Input: part model. Units: mm. Frame: model coordinates. A direction names the side the tool comes from. Round coordinates to 2 decimals unless told otherwise and drop trailing zeros. Loops run counter-clockwise (first coordinate to the right, second up) from the corner with the lowest first, then second, coordinate; pieces in that order, holes last. Notation, with made-up numbers: (32.25, 14) -> (89.25, 14) arc R14 cw to (89.25, 37) -> close; hole circle Ø7 at (29, 65). An arc over 180 degrees is marked (long way). Answer as a JSON object with one key per item and string values.
Autodesk Inventor part; units mm, degrees
ref_plane "YZ Plane" through (0, 0, 0) normal (1, 0, 0) x (0, 1, 0)
ref_plane "XY Plane" through (0, 0, 0) normal (0, 0, 1) x (1, 0, 0)
sketch "Sketch1" plane through (0, 0, 0) normal (0, 1, 0) x (-1, 0, 0)
  arc A0 (24.5855, 23.6396) -> (8.8578, 61.8356) centre (-39.8212, 19.4554) ccw
  arc A1 (8.8578, 61.8356) -> (-24.5592, 49.0787) centre (-2.8694, 42.4084) ccw
  arc A2 (-27.4284, -51.6159) -> (7.5457, -75.9974) centre (10.0017, -35.1993) ccw
  arc A3 (7.5457, -75.9974) -> (24.5855, 23.6396) centre (-254.8198, 20.1477) ccw
  arc A4 (21.8724, 23.5336) -> (7.0955, 59.7239) centre (-39.8212, 19.4554) ccw
  arc A5 (7.0955, 59.7239) -> (-21.8846, 48.5356) centre (-2.8694, 42.4084) ccw
  arc A6 (-21.8846, -56.1581) -> (5.7032, -73.1142) centre (10.0017, -35.1993) ccw
  arc A7 (5.7032, -73.1142) -> (21.8724, 23.5336) centre (-254.8198, 20.1477) ccw
  line L0 (-21.8846, 48.5356) -> (-21.8846, -56.1581)
  line L1 (-24.5592, 49.0787) -> (-27.4313, -51.6092)
  arc A8 (24.5855, 23.6396) -> (8.8578, 61.8356) centre (-39.8212, 19.4554) ccw
  arc A9 (8.8578, 61.8356) -> (-24.5592, 49.0787) centre (-2.8694, 42.4084) ccw
  arc A10 (-27.4313, -51.6092) -> (7.5457, -75.9974) centre (10.0017, -35.1993) ccw
  arc A11 (7.5457, -75.9974) -> (24.5855, 23.6396) centre (-254.8198, 20.1477) ccw
  line L2 (-24.5592, 49.0787) -> (-27.4313, -51.6092)
  point P0 (0, 0)
extrude "Extrusion1" add sketch "Sketch1" along normal blind 15.24
sketch "Sketch2" plane through (0, 0, 0) normal (0, 1, 0) x (-1, 0, 0)
  arc A0 (21.8724, 23.5336) -> (7.0955, 59.7239) centre (-39.8212, 19.4554) ccw
  arc A1 (5.7032, -73.1142) -> (21.8724, 23.5336) centre (-254.8198, 20.1477) ccw
  arc A2 (-21.8846, -56.1581) -> (5.7032, -73.1142) centre (10.0017, -35.1993) ccw
  line L0 (-21.8846, -56.1581) -> (-21.8846, 48.5356)
  arc A3 (7.0955, 59.7239) -> (-21.8846, 48.5356) centre (-2.8694, 42.4084) ccw
  arc A4 (20.2233, 23.4688) -> (6.03, 58.4313) centre (-39.8212, 19.4554) ccw
  arc A5 (6.03, 58.4313) -> (-20.235, 48.2707) centre (-2.8694, 42.4084) ccw
  line L1 (-20.235, 48.2707) -> (-20.235, -55.6586)
  arc A6 (-20.235, -55.6586) -> (4.5953, -71.3048) centre (10.0017, -35.1993) ccw
  arc A7 (4.5953, -71.3048) -> (20.2233, 23.4688) centre (-254.8198, 20.1477) ccw
  arc A8 (21.96, 23.537) -> (7.1522, 59.7924) centre (-39.8212, 19.4554) ccw
  arc A9 (7.1522, 59.7924) -> (-21.9723, 48.5494) centre (-2.8694, 42.4084) ccw
  line L2 (-21.9723, 48.5494) -> (-21.9723, -56.1844)
  arc A10 (-21.9723, -56.1844) -> (5.7624, -73.209) centre (10.0017, -35.1993) ccw
  arc A11 (5.7624, -73.209) -> (21.96, 23.537) centre (-254.8198, 20.1477) ccw
  point P0 (0, 0)
ref_plane "Work Plane2" through (0, 7.62, 0) normal (0, 1, 0) x (-1, 0, 0)
sketch "Sketch3" plane through (0, 7.62, 0) normal (0, 1, 0) x (-1, 0, 0)
  arc A0 (21.8724, 23.5336) -> (7.0955, 59.7239) centre (-39.8212, 19.4554) ccw
  arc A1 (5.7032, -73.1142) -> (21.8724, 23.5336) centre (-254.8198, 20.1477) ccw
  arc A2 (-21.8846, -56.1581) -> (5.7032, -73.1142) centre (10.0017, -35.1993) ccw
  arc A3 (5.7032, -73.1142) -> (21.8724, 23.5336) centre (-254.8198, 20.1477) ccw
  arc A4 (-21.8846, -56.1581) -> (5.7032, -73.1142) centre (10.0017, -35.1993) ccw
  line L0 (-21.8846, -56.1581) -> (-21.8846, 48.5356)
  arc A5 (7.0955, 59.7239) -> (-21.8846, 48.5356) centre (-2.8694, 42.4084) ccw
  arc A6 (21.8724, 23.5336) -> (7.0955, 59.7239) centre (-39.8212, 19.4554) ccw
  arc A7 (8.8578, 61.8356) -> (-24.5592, 49.0787) centre (-2.8694, 42.4084) ccw
  line L1 (-24.5592, 49.0787) -> (-27.4313, -51.6092)
  arc A8 (-27.4313, -51.6092) -> (7.5457, -75.9974) centre (10.0017, -35.1993) ccw
  arc A9 (7.5457, -75.9974) -> (24.5855, 23.6396) centre (-254.8198, 20.1477) ccw
  arc A10 (24.5855, 23.6396) -> (8.8578, 61.8356) centre (-39.8212, 19.4554) ccw
  arc A11 (20.0927, 23.4636) -> (5.7444, 58.5644) centre (-39.8212, 19.4554) ccw
  arc A12 (4.508, -71.1594) -> (20.0927, 23.4636) centre (-254.8198, 20.1477) ccw
  arc A13 (-20.3969, -55.1802) -> (4.508, -71.1594) centre (10.0017, -35.1993) ccw
  line L2 (-20.0973, 48.248) -> (-20.0973, -55.6163)
  arc A14 (-20.0973, -55.6163) -> (4.5033, -71.1517) centre (10.0017, -35.1993) ccw
  arc A15 (4.5033, -71.1517) -> (20.0858, 23.4633) centre (-254.8198, 20.1477) ccw
  arc A16 (20.0858, 23.4633) -> (5.9414, 58.323) centre (-39.8212, 19.4554) ccw
  arc A17 (5.9414, 58.323) -> (-20.0973, 48.248) centre (-2.8694, 42.4084) ccw
  arc A18 (21.9213, 23.5355) -> (7.1272, 59.7622) centre (-39.8212, 19.4554) ccw
  arc A19 (5.7363, -73.1672) -> (21.9213, 23.5355) centre (-254.8198, 20.1477) ccw
  arc A20 (-21.9336, -56.1728) -> (5.7363, -73.1672) centre (10.0017, -35.1993) ccw
  line L3 (-21.9336, -56.1728) -> (-21.9336, 48.5433)
  arc A21 (7.1272, 59.7622) -> (-21.9336, 48.5433) centre (-2.8694, 42.4084) ccw
  point P0 (0, 0)
extrude "Extrusion2" add sketch "Sketch3" along normal mid plane 5.08 contours A1 A2 L0 A5 A0
properties part number "track" material "PBT Plastic"
1) Reachability of faces 5 (the face through (9.641, 7.584, 59.292)), 6 (the face through (10.296, 12.664, 60.955)), 7 (the face through (-18.213, 2.504, -24.831)) from +Z, -Z, +X, -X, +Y, -Y: full face, straight path, thin tool, end or side. Return the list, or none.
Output:
{"face 5": "+Y, -Y", "face 6": "+Y", "face 7": "-Y"}
2) Draft query along Z for faces 1 (the face through (21, 5.08, -5)), 2 (the face through (-19.75, 7.51, 44.3)), 3 (the face through (13.11, 7.51, -68.91)), 4 (the face through (23, 15.24, 0)). Return one class per face: +Z half, -Z half, draft (parallel to the pull), parting line (faces both ways), or undercut.
Output:
{"face 1": "undercut", "face 2": "+Z half", "face 3": "-Z half", "face 4": "draft"}
3) Contact query for flat-ended pins moving along their axis: P1, Ø2.5, axis at y = 7, z = 18.5, coming from the -X side; P2, Ø2, axis at x = 22, y = 11, coming from the -Z side; P3, Ø3, axis at y = 3, z = -0.5, coming from the -X side. Output: stop coordinate, or through.
Output:
{"P1": "stops at x = -24.61", "P2": "stops at z = -61.83", "P3": "stops at x = -23.95"}
4) Section B-B, the plane z = 10. Output: boundary loops of the cut face in (x, y), plus the area to 3 significant figures.
Output:
{"outline": "(-24.42, 0) -> (-21.71, 0) -> (-21.71, 5.08) -> (-19.92, 5.08) -> (-19.92, 10.16) -> (-21.71, 10.16) -> (-21.71, 15.24) -> (-24.42, 15.24) -> close; (20.1, 5.08) -> (21.88, 5.08) -> (21.88, 0) -> (25.67, 0) -> (25.67, 15.24) -> (21.88, 15.24) -> (21.88, 10.16) -> (20.1, 10.16) -> close", "area": "117 mm^2"}
5) Section C-C, the plane x = 16.5. Output: boundary loops of the cut face in (y, z), plus the area to 3 significant figures.
Output:
{"outline": "(0, -66.31) -> (15.24, -66.31) -> (15.24, -62.65) -> (10.16, -62.65) -> (10.16, -60.11) -> (5.08, -60.11) -> (5.08, -62.65) -> (0, -62.65) -> close; (0, 57.01) -> (5.08, 57.01) -> (5.08, 54.45) -> (10.16, 54.45) -> (10.16, 57.01) -> (15.24, 57.01) -> (15.24, 60.55) -> (0, 60.55) -> close", "area": "136 mm^2"}
6) Ray query, probe 1 along Y at (x, z) = (21, 16); probe 2 along Z at (x, y) = (4, 14.75); probe 3 along Z at (x, y) = (-3, 2.25). Return the intervals inside material, ascending.
Output:
{"probe 1": "y = 5.08 to 10.16", "probe 2": "z = -73.6 to -70.7, 62.35 to 65.07", "probe 3": "z = -75.47 to -72.71, 61.5 to 64.33"}
